CAD build for the part. Positions are in the model's coordinates, mm. Give positions to 0.01 mm unless a question says otherwise; leave off trailing zeros. Write each loop counter-clockwise with the first axis right and the second up, starting at its lowest first coordinate (ties: lowest second). Pieces come first, ordered by that corner, then holes. Notation, with made-up numbers: (-18.75, 47) - (24.25, 47) arc R22 ccw to (24.25, 78) - close; hole circle Ø9 at (23.5, 5.5). An arc over 180 degrees is marked (long way). Put each result on its own line as item: value. Start each with the question number.
1. Cut at D-D on x = 68. List the corners of the cut face in (y, z), and give its area (3 significant figures).
2. Cut at B-B on z = 139. List the corners of the cut face in (x, y), and give its area (3 significant figures).
3. Mould opens along X. For faces 1 (the flat face through (70.64, 19.32, 139.52)), 2 (the flat face through (101.6, 19, 75)), 3 (the flat face through (41.52, 19.32, 139.88)), 4 (the flat face through (57, 38.1, 75)) say: +X half, -X half, draft (parallel to the pull), parting line (faces both ways), or undercut.
4. Cut at A-A on y = 36.5. List the corners of the cut face in (x, z), and give its area (3 significant figures).
5. Drop a flat-ended pin along its axis: pin 1 (1 mm diameter, centred on x = 74.5, y = 20, fed in from +Z). Give the stop position or say it passes through.
6. Wall check: line 1 (X direction, y = 27, z = 133.5); line 2 (Z direction, x = 86, y = 33.5); line 3 (Z direction, x = 46.5, y = 21). Give the ranges that are in metal, low to high.
7. Cut at C-C on x = 87. List the corners of the cut face in (y, z).
from build123d import *

# Parameters (mm, degrees)
SKETCH2_W               = 101.6
SKETCH2_H               = 50.8
BOSS_EXTRUDE1_DEPTH     = 152.4
CUT_EXTRUDE1_DEPTH      = 191.076195248
CUT_EXTRUDE1_DEPTH_BACK = 191.076195248
CUT_EXTRUDE2_DEPTH      = 191.076195248
CUT_EXTRUDE2_DEPTH_BACK = 191.076195248
SKETCH4_W               = 67.31
SKETCH4_H               = 12.7


with BuildPart() as part:
    # Sketch2 → Boss-Extrude1 (new body)
    with BuildSketch(Plane.XY):
        with Locations((50.8, 25.4)):
            Rectangle(SKETCH2_W, SKETCH2_H)
    extrude(amount=BOSS_EXTRUDE1_DEPTH)

    # Sketch3 → Cut-Extrude1 (cut, two sides: drawn at the far end of the back side and taken through both)
    with BuildSketch(Plane.XZ.offset(-CUT_EXTRUDE1_DEPTH_BACK)):
        Polygon((-149.218366946, 470.245815165), (34.29, 152.4), (48.954696837, 127), (92.94878735, 152.4), (410.794602514, 335.908366946), (582.019022435, 1049.69217865), (22.006052975, 1184.029626869), align=None)
    extrude(amount=CUT_EXTRUDE1_DEPTH + CUT_EXTRUDE1_DEPTH_BACK, mode=Mode.SUBTRACT)

    # Sketch4 → Cut-Extrude2 (cut, two sides: drawn at the far end of the back side and taken through both)
    with BuildSketch(Plane.XY.offset(152.4).offset(-CUT_EXTRUDE2_DEPTH_BACK)):
        Polygon((0, 0), (12.7, 0), (12.7, 38.1), (34.29, 38.1), (34.29, 50.8), (0, 50.8), align=None)
        with Locations((67.945, 44.45)):
            Rectangle(SKETCH4_W, SKETCH4_H)
    extrude(amount=CUT_EXTRUDE2_DEPTH + CUT_EXTRUDE2_DEPTH_BACK, mode=Mode.SUBTRACT)


solid = part.part
Report:
1. outline: (0, 0) - (38.1, 0) - (38.1, 138) - (0, 138) - close
1. area: 5,260 mm²
2. outline: (12.7, 0) - (42.03, 0) - (42.03, 38.1) - (12.7, 38.1) - close; (69.74, 0) - (101.6, 0) - (101.6, 38.1) - (69.74, 38.1) - close
2. area: 2,330 mm²
3. face 1: undercut
3. face 2: +X half
3. face 3: undercut
3. face 4: draft
4. outline: (12.7, 0) - (101.6, 0) - (101.6, 152.4) - (92.95, 152.4) - (48.95, 127) - (34.29, 152.4) - (12.7, 152.4) - close
4. area: 12,800 mm²
5. pin 1: stops at z = 142.04
6. line 1: x = 12.7 to 45.2, 60.21 to 101.6
6. line 2: z = 0 to 148.39
6. line 3: z = 0 to 131.25
7. outline: (0, 0) - (38.1, 0) - (38.1, 148.97) - (0, 148.97) - close
